Design review of the part built by this model. Coordinates are the model's own, in mm. A direction names the side the tool comes from. Round coordinates to 2 decimals unless told otherwise and drop trailing zeros. Write each loop counter-clockwise with the first axis right and the second up, starting at its lowest first coordinate (ties: lowest second). Pieces come first, ordered by that corner, then holes. Notation, with made-up numbers: (-3.5, 29.25) -> (6.5, 29.25) arc R33 ccw to (6.5, 58.25) -> close; hole circle Ø11 at (-21, -9.75). An arc over 180 degrees is marked (long way). One line per question, with ' | ' between items. Start each with the question number.
1) Mouldability with a two-part tool opening along Y and no side actions: class faces 1 (the flat face through (-3, 0, 13)), 2 (the flat face through (14.685, -14.378, 12.522)), 3 (the cylindrical face through (1.387, -1.306, 12.522)) as +Y half, -Y half, draft (parallel to the pull), parting line (faces both ways), or undercut.
2) Consider section B-B (y = -14). Give the boundary of the cut face in (x, z).
3) Insertion check: pin 1 Ø2 at (x, z) = (-1, 13) entering from -Y; pin 2 Ø1 at (x, y) = (13, -4) entering from -Z; pin 3 Ø0.7 at (x, z) = (-3, 17) entering from +Y. Each pin has a flat end and moves straight along its axis. Give the tip position at first contact, or say it passes through.
4) Consider section C-C (y = 1). Give the boundary of the cut face in (x, z), then the cut area to 3 significant figures.
5) For probe 1 along Y at (x, z) = (1, 20); probe 2 along Y at (x, z) = (1.75, 13.5); probe 3 along X at (y, z) = (-13.5, 20.25), list the stretches that pass through material, from the lowest coordinate up.
6) For faces 4 (the flat face through (0, 3, 13)), 5 (the cylindrical face through (-3.72, -0.83, 12.52)), 6 (the flat face through (1.65, -27.35, 12.52)), list the 3-axis set-ups (+Z, -Z, +X, -X, +Y, -Y) from which the entire face can be reached by the end or side of a thin tool; tool diameter is ignored.
7) Consider section A-A (z = 17.5). Give the boundary of the cut face in (x, y) (3 decimals).
```python
from build123d import *

# Parameters (mm, degrees)
F1_DEPTH    = 25.4
F3_DEPTH    = 25.4
F4_T1_DEPTH = 37.28706828
F5_T1_DEPTH = 27.7495122548


# Not quite as in the source:
# - a fillet or chamfer that OpenCascade refuses, or shapes differently, is made with other operations: its cross-section is extruded or revolved along the edge and cut away or added


with BuildPart() as f1:
    # F0 (on Top) → F1 (new body)
    with BuildSketch(Plane.XY):
        with BuildLine():
            ThreePointArc((0, 1.905), (1.3470384182, -1.3470384182), (-1.905, 0))
            Line((-1.905, 0), (-3.81, 0))
            ThreePointArc((-3.81, 0), (2.6940768363, -2.6940768363), (0, 3.81))
            Line((0, 3.81), (0, 1.905))
        make_face()
    extrude(amount=F1_DEPTH)

    # F2 (on face) → F3 (join)
    with BuildSketch(Plane.XY.offset(25.4)):
        with BuildLine():
            ThreePointArc((3.1994926084, -2.0686582726), (2.9633304397, -2.3947385463), (2.6940768363, -2.6940768363))
            Line((2.6940768363, -2.6940768363), (2.6940768363, -4.4720768363))
            ThreePointArc((2.6940768363, -4.4720768363), (10.4170971004, -7.6710565722), (13.6160768363, -15.3940768363))
            Line((13.6160768363, -15.3940768363), (16.0290768363, -15.3940768363))
            ThreePointArc((16.0290768363, -15.3940768363), (14.6027952108, -9.393689209), (10.6290540875, -4.6768775275))
            ThreePointArc((10.6290540875, -4.6768775275), (7.1111754901, -2.8118884542), (3.1994926084, -2.0686582726))
        make_face()
        with BuildLine():
            Line((2.5200781238, 2.8575), (2.6649185174, 2.7229229323))
            ThreePointArc((2.6649185174, 2.7229229323), (2.5933714137, 2.7911511444), (2.5200781238, 2.8575))
        make_face()
        with BuildLine():
            Line((2.6940768363, -4.4720768363), (2.6940768363, -2.6940768363))
            ThreePointArc((2.6940768363, -2.6940768363), (0.2570925649, -3.8013160107), (-2.3067877079, -3.0322978862))
            ThreePointArc((-2.3067877079, -3.0322978862), (-4.1681303207, -3.9602525446), (-5.862543163, -5.1663459449))
            ThreePointArc((-5.862543163, -5.1663459449), (-9.840056888, -19.9457487029), (2.6940768363, -28.7290768363))
            Line((2.6940768363, -28.7290768363), (2.6940768363, -26.3160768363))
            ThreePointArc((2.6940768363, -26.3160768363), (-8.2279231637, -15.3940768363), (2.6940768363, -4.4720768363))
        make_face()
        with BuildLine():
            ThreePointArc((2.6649185174, 2.7229229323), (3.7865078996, 0.4224428078), (3.1994926084, -2.0686582726))
            ThreePointArc((3.1994926084, -2.0686582726), (7.1111754901, -2.8118884542), (10.6290540875, -4.6768775275))
            Line((10.6290540875, -4.6768775275), (2.6649185174, 2.7229229323))
        make_face()
        with BuildLine():
            ThreePointArc((-5.862543163, -5.1663459449), (-4.1681303207, -3.9602525446), (-2.3067877079, -3.0322978862))
            ThreePointArc((-2.3067877079, -3.0322978862), (-2.9573260731, -2.4021495576), (-3.4407495541, -1.6362586916))
            Line((-3.4407495541, -1.6362586916), (-5.862543163, -5.1663459449))
        make_face()
    extrude(amount=-F3_DEPTH)

    # F4: chamfer of 2.54 on 2 edges, made by hand

    # F4_s2 → F4_t1 (cut)
    with BuildSketch(Plane.XY.offset(-5.94353414)):
        with BuildLine():
            Line((0.6333221193, -26.1199042634), (2.6940768363, -28.6142827349))
            Line((2.6940768363, -28.6142827349), (2.6940768363, -26.3160768363))
            ThreePointArc((2.6940768363, -26.3160768363), (1.6230071606, -26.2634325555), (0.6333221193, -26.1199042634))
        make_face()
        with BuildLine():
            Line((15.9142827349, -15.3940768363), (13.4199042634, -13.3333221193))
            ThreePointArc((13.4199042634, -13.3333221193), (13.5634325555, -14.3230071606), (13.6160768363, -15.3940768363))
            Line((13.6160768363, -15.3940768363), (15.9142827349, -15.3940768363))
        make_face()
    extrude(amount=F4_T1_DEPTH, mode=Mode.SUBTRACT)

    # F5: chamfer of 0.508 on 2 edges, made by hand

    # F5_s2 → F5_t1 (cut)
    with BuildSketch(Plane.XY.offset(-1.1747561274)):
        with BuildLine():
            Line((-1.8623055031, -0.4010526316), (-2.3589203039, 0))
            Line((-2.3589203039, 0), (-1.905, 0))
            ThreePointArc((-1.905, 0), (-1.8935148697, -0.2088694284), (-1.8623055031, -0.4010526316))
        make_face()
        with BuildLine():
            Line((0.4010526316, 1.8623055031), (0, 2.3589203039))
            Line((0, 2.3589203039), (0, 1.905))
            ThreePointArc((0, 1.905), (0.2088694284, 1.8935148697), (0.4010526316, 1.8623055031))
        make_face()
    extrude(amount=F5_T1_DEPTH, mode=Mode.SUBTRACT)


solid = f1.part
```
From the geometry:
1) face 1: +Y half | face 2: -Y half | face 3: undercut
2) outline: (-10.57, 0) -> (-8.14, 0) -> (-8.14, 25.4) -> (-10.57, 25.4) -> close; (14.23, 0) -> (15.96, 0) -> (15.96, 25.4) -> (14.23, 25.4) -> close
3) pin 1: stops at y = -28.45 | pin 2: passes through | pin 3: stops at y = 0
4) outline: (1.62, 0) -> (4.52, 0) -> (4.52, 25.4) -> (1.62, 25.4) -> close | area: 73.6 mm2
5) probe 1: y = -28.62 to -26.56, -4.6 to -1.62, 1.62 to 3.68 | probe 2: y = -28.7 to -27.47, -4.51 to -0.75, 0.75 to 3.38 | probe 3: x = -10.51 to -8.06, 13.62 to 15.89
6) face 4: +Z, -Z, -X, +Y | face 5: +Z, -Z, -X | face 6: +Z, -Z, +X
7) outline: (-5.863, -5.166) arc R13.335 ccw to (2.694, -28.729) -> (2.694, -28.614) -> (0.633, -26.12) arc R10.922 cw (long way) to (13.42, -13.333) -> (15.914, -15.394) -> (16.029, -15.394) arc R13.335 ccw to (10.629, -4.677) -> (2.665, 2.723) arc R3.81 ccw to (0, 3.81) -> (0, 2.359) -> (0.401, 1.862) arc R1.905 cw (long way) to (-1.862, -0.401) -> (-2.359, 0) -> (-3.81, 0) arc R3.81 ccw to (-3.441, -1.636) -> close
